from build123d import *


with BuildPart() as part:
    # Sketch2 → Revolve1 (revolve)
    with BuildSketch(Plane(origin=(0, 0, 0), x_dir=(1, 0, 0), z_dir=(0, 1, 0))):
        Polygon((0, 0), (0, 67), (-5, 67), (-5, 63), (-3, 63), (-3, 61), (-5, 61), (-5, 41.5), (-3, 41.5), (-3, 39.5), (-5, 39.5), (-5, 27.5), (-3, 27.5), (-3, 25.5), (-5, 25.5), (-5, 6), (-3, 6), (-3, 4), (-5, 4), (-5, 0), align=None)
    revolve(axis=Axis((0, 0, -67), (0, 0, 1)))


solid = part.part
Verification items for the finished model (mm, model axes). A direction names the side the tool comes from. Give positions to 0.01 mm unless a question says otherwise; leave off trailing zeros. Loops run counter-clockwise (first coordinate to the right, second up) from the corner with the lowest first, then second, coordinate; pieces in that order, holes last.
1. Cross-section at A-A on y = -4. Record the cut outline in (x, z).
Derived:
outline: (-3, -67) - (3, -67) - (3, -63) - (-3, -63) - close; (-3, -61) - (3, -61) - (3, -41.5) - (-3, -41.5) - close; (-3, -39.5) - (3, -39.5) - (3, -27.5) - (-3, -27.5) - close; (-3, -25.5) - (3, -25.5) - (3, -6) - (-3, -6) - close; (-3, -4) - (3, -4) - (3, 0) - (-3, 0) - close
2. Release check for a two-part mould opening along Z. For faces 3 (the flat face through (0, 0, 0)), 4 (the flat face through (3.3, -0.1, -61)), 5 (the flat face through (-3.3, -0.1, -6)), 6 (the cylindrical face through (1.08, 4.88, -33.42)) record: +Z half, -Z half, draft (parallel to the pull), parting line (faces both ways), or undercut.
Derived:
face 3: +Z half
face 4: undercut
face 5: undercut
face 6: draft
3. Cross-section at B-B on x = -3.75. Record the cut outline in (y, z).
Derived:
outline: (-3.31, -67) - (3.31, -67) - (3.31, -63) - (-3.31, -63) - close; (-3.31, -61) - (3.31, -61) - (3.31, -41.5) - (-3.31, -41.5) - close; (-3.31, -39.5) - (3.31, -39.5) - (3.31, -27.5) - (-3.31, -27.5) - close; (-3.31, -25.5) - (3.31, -25.5) - (3.31, -6) - (-3.31, -6) - close; (-3.31, -4) - (3.31, -4) - (3.31, 0) - (-3.31, 0) - close
4. Tool access check on faces 1 (the flat face through (0, 0, -67)), 2 (the flat face through (3.3, -0.1, -4)). Record the directions out of +Z, -Z, +X, -X, +Y, -Y that give a thin tool (end or side, any length) a straight path to the whole face; none if there is none.
Derived:
face 1: -Z, +X, -X, +Y, -Y
face 2: none
5. Go/stop test with flat-tipped pins: P1, Ø3, axis at y = 3.5, z = -48.5, coming from the -X side; P2, Ø5, axis at x = -1.5, y = 2, coming from the +Z side; P3, Ø1, axis at x = -3.5, z = -53.5, coming from the -Y side. Record where each tip stops, or that it passes through.
Derived:
P1: stops at x = -4.58
P2: stops at z = 0
P3: stops at y = -4
6. Material ranges on probe 1 along Z at (x, y) = (-1.75, -4.25); probe 2 along Y at (x, z) = (4, -7.5); probe 3 along X at (y, z) = (-0.25, -28.5), recorded low to high.
Derived:
probe 1: z = -67 to -63, -61 to -41.5, -39.5 to -27.5, -25.5 to -6, -4 to 0
probe 2: y = -3 to 3
probe 3: x = -4.99 to 4.99
7. Cross-section at C-C on z = -17.5. Record the cut outline in (x, y), and give its area (3 significant figures).
Derived:
outline: circle Ø10 at (0, 0)
area: 78.5 mm2
